from build123d import *

# Parameters (mm, degrees)
SKETCH1_R           = 1.75
SKETCH1_R_2         = 1.5
BOSS_EXTRUDE1_DEPTH = 4.5


with BuildPart() as part:
    # Sketch1 → Boss-Extrude1 (new body)
    with BuildSketch(Plane(origin=(0, 0, 0), x_dir=(1, 0, 0), z_dir=(0, 1, 0))):
        with BuildLine():
            Line((-35.7, -55), (49.7, -55))
            ThreePointArc((49.7, -55), (53.942640687, -53.242640687), (55.7, -49))
            Line((55.7, -49), (55.7, -42.377818725))
            ThreePointArc((55.7, -42.377818725), (54.797249664, -39.212689049), (52.36065138, -37))
            Line((52.36065138, -37), (45.03934862, -33.377818725))
            ThreePointArc((45.03934862, -33.377818725), (42.602750336, -31.165129675), (41.7, -28))
            Line((41.7, -28), (41.7, 28))
            ThreePointArc((41.7, 28), (42.602750336, 31.165129675), (45.03934862, 33.377818725))
            Line((45.03934862, 33.377818725), (52.36065138, 37))
            ThreePointArc((52.36065138, 37), (54.797249664, 39.212689049), (55.7, 42.377818725))
            Line((55.7, 42.377818725), (55.7, 49))
            ThreePointArc((55.7, 49), (53.942640687, 53.242640687), (49.7, 55))
            Line((49.7, 55), (-63.3, 55))
            ThreePointArc((-63.3, 55), (-67.542640687, 53.242640687), (-69.3, 49))
            Line((-69.3, 49), (-69.3, 23.31729281))
            ThreePointArc((-69.3, 23.31729281), (-68.03372658, 19.630582533), (-64.769389112, 17.5))
            Line((-64.769389112, 17.5), (-46.230610888, 12.81729281))
            ThreePointArc((-46.230610888, 12.81729281), (-42.96627342, 10.686710277), (-41.7, 7))
            Line((-41.7, 7), (-41.7, -49))
            ThreePointArc((-41.7, -49), (-39.942640687, -53.242640687), (-35.7, -55))
        make_face()
        with Locations(Location((-63.8, 49.5, 0), (0, 0, 270))):
            Circle(SKETCH1_R, mode=Mode.SUBTRACT)
        with Locations(Location((-36.2, -49.5, 0), (0, 0, 270))):
            Circle(SKETCH1_R, mode=Mode.SUBTRACT)
        with Locations(Location((50.2, -49.5, 0), (0, 0, 270))):
            Circle(SKETCH1_R, mode=Mode.SUBTRACT)
        with Locations(Location((50.2, 49.5, 0), (0, 0, 270))):
            Circle(SKETCH1_R, mode=Mode.SUBTRACT)
        with Locations(Location((-10, 24.318057397, 0), (0, 0, 270))):
            Circle(SKETCH1_R, mode=Mode.SUBTRACT)
        with Locations(Location((-10, 4.318057397, 0), (0, 0, 270))):
            Circle(SKETCH1_R, mode=Mode.SUBTRACT)
        with Locations(Location((10, 4.318057397, 0), (0, 0, 270))):
            Circle(SKETCH1_R, mode=Mode.SUBTRACT)
        with Locations(Location((10, 24.318057397, 0), (0, 0, 270))):
            Circle(SKETCH1_R, mode=Mode.SUBTRACT)
        with Locations(Location((0, -25.681942603, 0), (0, 0, 270))):
            Circle(SKETCH1_R_2, mode=Mode.SUBTRACT)
    extrude(amount=BOSS_EXTRUDE1_DEPTH)


solid = part.part
Here's how the part is built. I have some questions about the finished solid (model axes, mm). A direction names the side the tool comes from. Round coordinates to 2 decimals unless told otherwise and drop trailing zeros. Write each loop counter-clockwise with the first axis right and the second up, starting at its lowest first coordinate (ties: lowest second). Pieces come first, ordered by that corner, then holes.
1. Suppose I cut it at A-A (x = 10). List the corners of the cut face in (y, z) for me, and give its area (4 significant figures).
2. If we mould it in two halves opening along X, with no side actions, what happens to faces 1 (the cylindrical face through (-67.496, 2.218, -53.289)), 2 (the cylindrical face through (-64.47, 2.218, -47.883)), 3 (the flat face through (48.751, 2.218, 35.214))? For each: released by +X, released by -X, zero draft, split by the parting line, or undercut.
3. For faces 4 (the cylindrical face through (-36.87, 2.218, 51.117)), 5 (the flat face through (48.649, 2.218, -35.164)), which set-ups out of +Z, -Z, +X, -X, +Y, -Y let a thin tool reach every point of the face, with its end or its side?
4. Suppose I cut it at C-C (z = -1). List the corners of the cut face in (x, y) for me, and give its area (3 significant figures).
5. Suppose I cut it at B-B (y = 2.8). State how many separate pieces and enclosed holes the cut face has, and give its area (3 significant figures).
6. I need wall thicknesses on L1, parallel to X at y = 2.15, z = 49.5; L2, parallel to Z at x = -36, y = 1.55; L3, parallel to Z at x = -1, y = 3.8. Which ranges of each line are inside material? Lowest first, please.
7. Will this pin go through, and if not, where does the flat tip stop? pin 1 Ø2 at (y, z) = (3.5, -23) entering from +X.
Answer sheet:
1. outline: (0, -55) - (4.5, -55) - (4.5, -26.07) - (0, -26.07) - close; (0, -22.57) - (4.5, -22.57) - (4.5, -6.07) - (0, -6.07) - close; (0, -2.57) - (4.5, -2.57) - (4.5, 55) - (0, 55) - close
1. area: 463.5 mm2
2. face 1: released by -X
2. face 2: undercut
2. face 3: released by +X
3. face 4: +Y, -Y
3. face 5: +X, +Y, -Y
4. outline: (-41.7, 0) - (41.7, 0) - (41.7, 4.5) - (-41.7, 4.5) - close
4. area: 375 mm2
5. separate pieces: 1
5. enclosed holes: 9
5. area: 10,700 mm2
6. L1: x = -41.68 to -37.95, -34.45 to 48.45, 51.95 to 55.68
6. L2: z = -55 to 47.76, 51.24 to 54.99
6. L3: z = -55 to 24.56, 26.8 to 55
7. pin 1: stops at x = 41.7
